```python
from build123d import *

# Parameters (mm, degrees)
SKETCH1_W           = 88.736
SKETCH1_H           = 25
SKETCH1_R           = 10.25
BOSS_EXTRUDE1_DEPTH = 3.2
FILLET1_R           = 3


with BuildPart() as part:
    # Sketch1 → Boss-Extrude1 (new body)
    with BuildSketch(Plane(origin=(0, 0, 0), x_dir=(1, 0, 0), z_dir=(0, 1, 0))):
        Rectangle(SKETCH1_W, SKETCH1_H)
        with Locations(Location((30.118, 0, 0), (0, 0, 270))):
            Circle(SKETCH1_R, mode=Mode.SUBTRACT)
        with Locations(Location((-30.118, 0, 0), (0, 0, 270))):
            Circle(SKETCH1_R, mode=Mode.SUBTRACT)
    extrude(amount=BOSS_EXTRUDE1_DEPTH)

    # Fillet1
    fillet1_edges = [part.edges().sort_by_distance(p)[0] for p in [
        (44.368, 1.6, -12.5),
        (44.368, 1.6, 12.5),
        (-44.368, 1.6, 12.5),
        (-44.368, 1.6, -12.5),
    ]]
    fillet(fillet1_edges, radius=FILLET1_R)


solid = part.part
```
Could you check a few things on this model? Use its own coordinates, in mm. Give positions to 0.01 mm unless a question says otherwise; leave off trailing zeros. Write each loop counter-clockwise with the first axis right and the second up, starting at its lowest first coordinate (ties: lowest second). Pieces come first, ordered by that corner, then holes. Notation, with made-up numbers: (87, 5) -> (131, 5) arc R27 cw to (131, 36) -> close; hole circle Ø4 at (75.25, 54). An arc over 180 degrees is marked (long way). Write each question's results on one line, items separated by ' | '.
1. I need wall thicknesses on L1, parallel to X at y = 2.4, z = 0; L2, parallel to X at y = 2.4, z = -6.5; L3, parallel to Z at x = 31, y = 1.15. Which ranges of each line are inside material? Lowest first, please.
Check sheet entries:
L1: x = -44.37 to -40.37, -19.87 to 19.87, 40.37 to 44.37 | L2: x = -44.37 to -38.04, -22.19 to 22.19, 38.04 to 44.37 | L3: z = -12.5 to -10.21, 10.21 to 12.5
2. I want a section at C-C, the plane y = 0.6. Write out the boundary of the cut face in (x, z), then the cut area to 3 significant figures.
Check sheet entries:
outline: (-44.37, -9.5) arc R3 ccw to (-41.37, -12.5) -> (41.37, -12.5) arc R3 ccw to (44.37, -9.5) -> (44.37, 9.5) arc R3 ccw to (41.37, 12.5) -> (-41.37, 12.5) arc R3 ccw to (-44.37, 9.5) -> close; hole circle Ø20.5 at (-30.12, 0); hole circle Ø20.5 at (30.12, 0) | area: 1,550 mm²
3. I want a section at A-A, the plane z = 0. Write out the boundary of the cut face in (x, y), then the cut area to 3 significant figures.
Check sheet entries:
outline: (-44.37, 0) -> (-40.37, 0) -> (-40.37, 3.2) -> (-44.37, 3.2) -> close; (-19.87, 0) -> (19.87, 0) -> (19.87, 3.2) -> (-19.87, 3.2) -> close; (40.37, 0) -> (44.37, 0) -> (44.37, 3.2) -> (40.37, 3.2) -> close | area: 153 mm²
4. I want a section at D-D, the plane x = 28.5. Write out the boundary of the cut face in (y, z).
Check sheet entries:
outline: (0, -12.5) -> (3.2, -12.5) -> (3.2, -10.12) -> (0, -10.12) -> close; (0, 10.12) -> (3.2, 10.12) -> (3.2, 12.5) -> (0, 12.5) -> close
5. I want a section at B-B, the plane x = -32.5. Write out the boundary of the cut face in (y, z), then the cut area to 3 significant figures.
Check sheet entries:
outline: (0, -12.5) -> (3.2, -12.5) -> (3.2, -9.97) -> (0, -9.97) -> close; (0, 9.97) -> (3.2, 9.97) -> (3.2, 12.5) -> (0, 12.5) -> close | area: 16.2 mm²
6. If we mould it in two halves opening along X, with no side actions, what happens to faces 1 (the flat face through (-1, 2, -12.5)), 2 (the flat face through (-44.368, 2, 0)), 3 (the cylindrical face through (38.76, 1.58, 5.51))? For each: released by +X, released by -X, zero draft, split by the parting line, or undercut.
Check sheet entries:
face 1: zero draft | face 2: released by -X | face 3: undercut
